from build123d import *

# Parameters (mm, degrees)
F0_R     = 7.5
F0_R_2   = 2.5
F1_DEPTH = 21
F2_R     = 10
F2_R_2   = 5.05
F3_DEPTH = 10
F5_D     = 2.7
F5_DEPTH = 10.001
F6_SIZE  = 0.5
F7_D     = 2.7


with BuildPart() as f1:
    # F0 (on Front) → F1 (new body)
    with BuildSketch(Plane.XZ):
        Circle(F0_R)
        Circle(F0_R_2, mode=Mode.SUBTRACT)
    extrude(amount=F1_DEPTH)

    # F2 (on Front) → F3 (join)
    with BuildSketch(Plane.XZ):
        Circle(F2_R)
        Circle(F2_R_2, mode=Mode.SUBTRACT)
    extrude(amount=-F3_DEPTH)

    # F5 (through all, one way)
    with BuildSketch(Plane.YZ):
        with Locations((5, 0), (-16, 0)):
            Circle(F5_D / 2)
    extrude(amount=-F5_DEPTH, mode=Mode.SUBTRACT)

    # F6
    f6_edges = [f1.edges().sort_by_distance(p)[0] for p in [
        (-10, 10, 0),
        (-5.05, 10, 0),
        (-10, 0, 0),
        (-7.5, -21, 0),
        (-2.5, -21, 0),
    ]]
    chamfer(f6_edges, length=F6_SIZE)

    # F7 (through all)
    with Locations(Plane(origin=(0, 0, 0), x_dir=(0, 1, 0), z_dir=(-1, 0, 0))):
        with Locations((5, 0), (-16, 0)):
            Hole(F7_D / 2)


solid = f1.part
Work out the finished part from the listing and answer in its coordinate system (mm). A direction names the side the tool comes from. Round coordinates to 2 decimals unless told otherwise and drop trailing zeros. Loops run counter-clockwise (first coordinate to the right, second up) from the corner with the lowest first, then second, coordinate; pieces in that order, holes last. Notation, with made-up numbers: (47.25, 3.5) - (68.25, 3.5) arc R29 cw to (68.25, 26.5) - close; hole circle Ø11 at (-9, 17.5). An arc over 180 degrees is marked (long way). One line per item, written item: value.
Q1. The mould has two halves that part along Z. Classify faces 3 (the cylindrical face through (6.93, -10.11, -2.87)), 4 (the cylindrical face through (-7.397, 6.247, -0.517)), 5 (the cylindrical face through (7.469, 3.712, -0.406)), 6 (the flat face through (1, 0, 8)): +Z half, -Z half, draft (parallel to the pull), parting line (faces both ways), or undercut.
Check values:
face 3: parting line
face 4: undercut
face 5: undercut
face 6: draft
Q2. Find section C-C on y = 5. Give the vertices of the cut face in (x, z).
Check values:
outline: (-9.91, -1.35) arc R10 ccw to (9.91, -1.35) - (4.87, -1.35) arc R5.05 cw to (-4.87, -1.35) - close; (-9.91, 1.35) - (-4.87, 1.35) arc R5.05 cw to (4.87, 1.35) - (9.91, 1.35) arc R10 ccw to start
Q3. For faces 1 (the flat face through (1, -21, -3)), 2 (the cylindrical face through (4.817, 4.684, 1.517)), determine the directions among +Z, -Z, +X, -X, +Y, -Y from which every point of the face is accessible in a straight line to the end or side of a thin tool.
Check values:
face 1: +Z, -Z, +X, -X, -Y
face 2: +Y
Q4. Straight lines are drawn through the part: probe 1 along X at (y, z) = (-11, 0); probe 2 along X at (y, z) = (2, 1). For each, find the intervals that lie inside material, in ascending order.
Check values:
probe 1: -7.5 to -2.5, 2.5 to 7.5
probe 2: -9.95 to -4.95, 4.95 to 9.95
Q5. Find section A-A on x = 0. Give the vertices of the cut face in (y, z).
Check values:
outline: (-21, -7) - (-20.5, -7.5) - (0, -7.5) - (0, -9.5) - (0.5, -10) - (9.5, -10) - (10, -9.5) - (10, -5.55) - (9.5, -5.05) - (0, -5.05) - (0, -2.5) - (-20.5, -2.5) - (-21, -3) - close; (-21, 3) - (-20.5, 2.5) - (0, 2.5) - (0, 5.05) - (9.5, 5.05) - (10, 5.55) - (10, 9.5) - (9.5, 10) - (0.5, 10) - (0, 9.5) - (0, 7.5) - (-20.5, 7.5) - (-21, 7) - close
Q6. Find section B-B on y = -6. Give the vertices of the cut face in (x, z), and give its area (3 significant figures).
Check values:
outline: circle Ø15 at (0, 0); hole circle Ø5 at (0, 0)
area: 157 mm2
Q7. Each of these flat-tipped pins is pushed along its axis until it touches: pin 1 Ø3 at (x, z) = (-0.5, 1.5) entering from +Y; pin 2 Ø1.5 at (y, z) = (-9, -1) entering from +X; pin 3 Ø2 at (x, y) = (-2, -5.5) entering from -Z. Where does it stop, or does it pass through?
Check values:
pin 1: y = 0
pin 2: x = 7.5
pin 3: z = -7.43
Q8. Find section D-D on z = 0. State how many separate pieces and enclosed holes the cut face has, and give its area (3 significant figures).
Check values:
separate pieces: 6
enclosed holes: 0
area: 254 mm2
